Check sheet for the modelled part. Datum: model origin and axes. Units: mm. A direction names the side the tool comes from. Give positions to 0.01 mm unless a question says otherwise; leave off trailing zeros. Write each loop counter-clockwise with the first axis right and the second up, starting at its lowest first coordinate (ties: lowest second). Pieces come first, ordered by that corner, then holes. Notation, with made-up numbers: (-17.5, 40.5) -> (2.5, 40.5) arc R27 cw to (2.5, 65.5) -> close; hole circle Ø7 at (52, 7). An arc over 180 degrees is marked (long way). Return JSON: item names as keys, results as strings.
Autodesk Inventor part; units mm, degrees
ref_plane "to_leaf1_XY" through (0, 1.9, 0) normal (0, 0, 1) x (1, 0, 0)
ref_plane "to_leaf1_YZ" through (0, 1.9, 0) normal (1, 0, 0) x (0, 1, 0)
ref_plane "to_leaf1_ZX" through (0, 1.9, 0) normal (0, 1, 0) x (0, 0, 1)
sketch "Sketch_15" plane through (0, 0, 0) normal (0, 0, 1) x (1, 0, 0)
  line L0 (-10, 0.8) -> (-10, 0)
  line L1 (-10, 0) -> (0, 0)
  arc A0 (0, 0) -> (-1.5492, 0.8) centre (0, 1.9) ccw
  line L2 (-1.5492, 0.8) -> (-10, 0.8)
  circle A1 centre (0, 1.9) radius 1
extrude "Extrusion1" add sketch "Sketch_15" against normal blind 25
sketch "Sketch_1" plane through (0, 0, 0) normal (0, 1, 0) x (-1, 0, 0)
  line L0 (2.09, -16.6667) -> (2.09, -8.3333)
  line L1 (2.09, -8.3333) -> (-2.09, -8.3333)
  line L2 (-2.09, -8.3333) -> (-2.09, 0)
  line L3 (-2.09, 0) -> (-6, 0)
  line L4 (-6, 0) -> (-6, -25)
  line L5 (-6, -25) -> (-2.09, -25)
  line L6 (-2.09, -25) -> (-2.09, -16.6667)
  line L7 (-2.09, -16.6667) -> (2.09, -16.6667)
extrude "Extrusion2" cut sketch "Sketch_1" along normal blind 3.8
sketch "Sketch3" plane through (-10, 0, 0) normal (0, -1, 0) x (1, 0, 0)
  point P0 (4, -20.5)
hole "Hole1" at (-6, 0, -20.5) direction (0, 1, 0) diameter 3.4 depth 0.8
pattern_linear "Rectangular Pattern1" count 2 spacing 16 along (0, 0, 1) of "Hole1"
ref_plane "to_leaf1_XY" through (0, 1.9, 0) normal (0, 0, 1) x (1, 0, 0)
ref_plane "to_leaf1_YZ" through (0, 1.9, 0) normal (1, 0, 0) x (0, 1, 0)
ref_plane "to_leaf1_ZX" through (0, 1.9, 0) normal (0, 1, 0) x (0, 0, 1)
properties part number "HHS25-LEAF2"
(1) Depth check by flat-ended pin: pin 1 Ø3 at (x, z) = (-6.5, -4) entering from +Y; pin 2 Ø1 at (x, y) = (-8, 1) entering from -Z. Enter the tip coordinate at first touch or a pass-through.
Reply:
{"pin 1": "y = 0.8", "pin 2": "z = -25"}
(2) Thickness scan on L1, parallel to Z at x = -6, y = 0.35; L2, parallel to Z at x = -0.25, y = 0.4; L3, parallel to Y at x = 0, z = -2.75. Record the ranges inside material, lowest first.
Reply:
{"L1": "-25 to -22.2, -18.8 to -6.2, -2.8 to 0", "L2": "-25 to -16.67, -8.33 to 0", "L3": "0 to 0.9, 2.9 to 3.8"}
(3) Release check for a two-part mould opening along X. For faces 3 (the cylindrical face through (-0.217, 0.924, -20.775)), 4 (the flat face through (-5, 0, -12)), 5 (the cylindrical face through (-4.5, 0.4, -5.3)) record: pulls with the +X half, pulls with the -X half, needs draft (parallel to the pull), parting line crosses it, or undercut.
Reply:
{"face 3": "undercut", "face 4": "needs draft", "face 5": "undercut"}
(4) Cross-section at C-C on x = -6. Enter the section's corners in (y, z), then the cut area to 3 significant figures.
Reply:
{"outline": "(0, -25) -> (0.8, -25) -> (0.8, -22.2) -> (0, -22.2) -> close; (0, -18.8) -> (0.8, -18.8) -> (0.8, -6.2) -> (0, -6.2) -> close; (0, -2.8) -> (0.8, -2.8) -> (0.8, 0) -> (0, 0) -> close", "area": "14.6 mm^2"}
(5) Set-up check for faces 1 (the cylindrical face through (-4.5, 0.4, -21.3)), 2 (the flat face through (-1, 1, -8.333)): record each of +Z, -Z, +X, -X, +Y, -Y from which the full face is reachable in a straight line by a thin tool's end or side.
Reply:
{"face 1": "+Y, -Y", "face 2": "+X, +Y, -Y"}
(6) Cross-section at D-D on z = -7. Enter the section's corners in (x, y).
Reply:
{"outline": "(-10, 0) -> (0, 0) arc R1.9 ccw (long way) to (-1.55, 0.8) -> (-10, 0.8) -> close; hole circle Ø2 at (0, 1.9)"}
(7) Cross-section at A-A on z = -20.5. Enter the section's corners in (x, y).
Reply:
{"outline": "(-10, 0) -> (-7.7, 0) -> (-7.7, 0.8) -> (-10, 0.8) -> close; (-4.3, 0) -> (0, 0) arc R1.9 ccw (long way) to (-1.55, 0.8) -> (-4.3, 0.8) -> close; hole circle Ø2 at (0, 1.9)"}
(8) Cross-section at B-B on y = 1.9. Enter the section's corners in (x, z), then the cut area to 3 significant figures.
Reply:
{"outline": "(-1.9, -25) -> (-1, -25) -> (-1, -16.67) -> (-1.9, -16.67) -> close; (-1.9, -8.33) -> (-1, -8.33) -> (-1, 0) -> (-1.9, 0) -> close; (1, -25) -> (1.9, -25) -> (1.9, -16.67) -> (1, -16.67) -> close; (1, -8.33) -> (1.9, -8.33) -> (1.9, 0) -> (1, 0) -> close", "area": "30.0 mm^2"}
